Check sheet for the modelled part. Datum: model origin and axes. Units: mm. Round coordinates to 2 decimals unless told otherwise and drop trailing zeros. Write each loop counter-clockwise with the first axis right and the second up, starting at its lowest first coordinate (ties: lowest second). Pieces come first, ordered by that corner, then holes. Notation, with made-up numbers: (8.5, 76.25) -> (64.5, 76.25) arc R6 cw to (64.5, 87.25) -> close; hole circle Ø5 at (48.25, 40.5). An arc over 180 degrees is marked (long way). One line per item, written item: value.
from build123d import *

# Parameters (mm, degrees)
ESQUISSE1_R                               = 53
BOSS_EXTRU_1_DEPTH                        = 5
CHANFREIN1_SIZE                           = 0.5
TROU_POUR_TARAUDAGE_POUR_TROU_TARAUD_M8_D = 6.8
CHANFREIN2_SIZE                           = 0.2
ESQUISSE4_R                               = 6
ENL_V_MAT_EXTRU_1_DEPTH                   = 76.119904153
CHANFREIN3_SIZE                           = 0.5


with BuildPart() as part:
    # Esquisse1 → Boss.-Extru.1 (new body)
    with BuildSketch(Plane.XY):
        Circle(ESQUISSE1_R)
    extrude(amount=BOSS_EXTRU_1_DEPTH)

    # Chanfrein1
    chanfrein1_edges = [part.edges().sort_by_distance(p)[0] for p in [
        (-53, 0, 0),
        (-53, 0, 5),
    ]]
    chamfer(chanfrein1_edges, length=CHANFREIN1_SIZE)

    # Trou pour taraudage pour trou taraudé M81 (through all)
    with Locations(Plane.XY.offset(5)):
        with Locations((0, 45.033320997), (39, -22.516660498), (-39, -22.516660498)):
            Hole(TROU_POUR_TARAUDAGE_POUR_TROU_TARAUD_M8_D / 2)

    # Chanfrein2
    chanfrein2_edges = [part.edges().sort_by_distance(p)[0] for p in [
        (-35.6, -22.516660498, 5),
        (-35.6, -22.516660498, 0),
        (42.4, -22.516660498, 5),
        (42.4, -22.516660498, 0),
        (3.4, 45.033320997, 5),
        (3.4, 45.033320997, 0),
    ]]
    chamfer(chanfrein2_edges, length=CHANFREIN2_SIZE)

    # Esquisse4 → Enlèv. mat.-Extru.1 (cut, through all)
    with BuildSketch(Plane.XY.offset(5)):
        Circle(ESQUISSE4_R)
    extrude(amount=-ENL_V_MAT_EXTRU_1_DEPTH, mode=Mode.SUBTRACT)

    # Chanfrein3
    chanfrein3_edges = [part.edges().sort_by_distance(p)[0] for p in [
        (-6, 0, 0),
    ]]
    chamfer(chanfrein3_edges, length=CHANFREIN3_SIZE)


solid = part.part
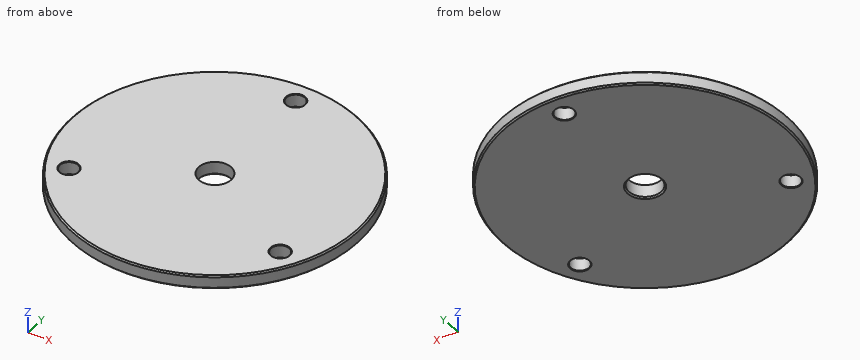
Item 1: Sectioned sample at B-B on x = 0. Enter the section's corners in (y, z).
Answer:
outline: (-53, 0.5) -> (-52.5, 0) -> (-6.5, 0) -> (-6, 0.5) -> (-6, 5) -> (-52.5, 5) -> (-53, 4.5) -> close; (6, 0.5) -> (6.5, 0) -> (41.43, 0) -> (41.63, 0.2) -> (41.63, 4.8) -> (41.43, 5) -> (6, 5) -> close; (48.43, 0.2) -> (48.63, 0) -> (52.5, 0) -> (53, 0.5) -> (53, 4.5) -> (52.5, 5) -> (48.63, 5) -> (48.43, 4.8) -> close
Item 2: Sectioned sample at D-D on y = -21. Count the separate pieces of the cut face and the enclosed holes in it, and give its area (3 significant figures).
Answer:
separate pieces: 3
enclosed holes: 0
area: 425 mm^2
Item 3: Sectioned sample at A-A on y = 0. Enter the section's corners in (x, z), and give its area (3 significant figures).
Answer:
outline: (-53, 0.5) -> (-52.5, 0) -> (-6.5, 0) -> (-6, 0.5) -> (-6, 5) -> (-52.5, 5) -> (-53, 4.5) -> close; (6, 0.5) -> (6.5, 0) -> (52.5, 0) -> (53, 0.5) -> (53, 4.5) -> (52.5, 5) -> (6, 5) -> close
area: 469 mm^2
Item 4: Depth check by flat-ended pin: P1, Ø6, axis at x = 39, y = -22.52, coming from the -Z side; P2, Ø3, axis at x = -2.5, z = 4, coming from the -Y side; P3, Ø2, axis at x = 40, z = 1, coming from the -Y side. Enter the tip coordinate at first touch or a pass-through.
Answer:
P1: passes through
P2: stops at y = -52.99
P3: stops at y = -35.89
Item 5: Sectioned sample at C-C on z = 3.15. Enter the section's corners in (x, y), and give its area (3 significant figures).
Answer:
outline: circle Ø106 at (0, 0); hole circle Ø6.8 at (-39, -22.52); hole circle Ø12 at (0, 0); hole circle Ø6.8 at (0, 45.03); hole circle Ø6.8 at (39, -22.52)
area: 8,600 mm^2
Item 6: Thickness scan on line 1 (Y direction, x = 0, z = 3.8); line 2 (X direction, y = -21, z = 3.75); line 3 (X direction, y = -5.5, z = 3.25). Record the ranges inside material, lowest first.
Answer:
line 1: y = -53 to -6, 6 to 41.63, 48.43 to 53
line 2: x = -48.66 to -42.04, -35.96 to 35.96, 42.04 to 48.66
line 3: x = -52.71 to -2.4, 2.4 to 52.71
